from build123d import *

# Parameters (mm, degrees)
CROQUIS1_R              = 1.625
CUERPO_INICIAL_DEPTH    = 2.5
SALIENTE_EXTRUIR2_DEPTH = 195
CROQUIS6_W              = 143
CROQUIS6_H              = 28
CORTAR_EXTRUIR1_DEPTH   = 10


with BuildPart() as part:
    # Croquis1 → Cuerpo Inicial (new body)
    with BuildSketch(Plane(origin=(0, 0, 0), x_dir=(1, 0, 0), z_dir=(0, 1, 0))):
        Polygon((-71.5, -25), (-71.5, -61), (71.5, -61), (71.5, -25), (97.5, -25), (97.5, 0), (97.5, 1), (97.5, 5.7), (45, 5.7), (-45, 5.7), (-97.5, 5.7), (-97.5, 1), (-97.5, 0), (-97.5, -25), align=None)
        with Locations((-92.5, -12)):
            Circle(CROQUIS1_R, mode=Mode.SUBTRACT)
        with Locations((-64, -12)):
            Circle(CROQUIS1_R, mode=Mode.SUBTRACT)
        with Locations((-92.5, -0.46)):
            Circle(CROQUIS1_R, mode=Mode.SUBTRACT)
        with Locations((-64, -0.46)):
            Circle(CROQUIS1_R, mode=Mode.SUBTRACT)
        with Locations((64, -12)):
            Circle(CROQUIS1_R, mode=Mode.SUBTRACT)
        with Locations((92.5, -12)):
            Circle(CROQUIS1_R, mode=Mode.SUBTRACT)
        with Locations((64, -0.46)):
            Circle(CROQUIS1_R, mode=Mode.SUBTRACT)
        with Locations((92.5, -0.46)):
            Circle(CROQUIS1_R, mode=Mode.SUBTRACT)
    extrude(amount=CUERPO_INICIAL_DEPTH)

    # Croquis3 → Saliente-Extruir2 (add)
    with BuildSketch(Plane(origin=(97.5, 0, 0), x_dir=(0, 0, -1), z_dir=(1, 0, 0))):
        Polygon((5.7, 2.5), (17.833199952, 2.5), (20.75, 0), (5.7, 0), align=None)
    extrude(amount=-SALIENTE_EXTRUIR2_DEPTH)

    # Croquis6 → Cortar-Extruir1 (cut)
    with BuildSketch(Plane(origin=(0, 2.5, 0), x_dir=(1, 0, 0), z_dir=(0, 1, 0))):
        with Locations((0, -47)):
            Rectangle(CROQUIS6_W, CROQUIS6_H)
    extrude(amount=-CORTAR_EXTRUIR1_DEPTH, mode=Mode.SUBTRACT)


solid = part.part
Source: CAD feature listing. Evaluate the final solid. Frame: model axes, mm. Round coordinates to 2 decimals unless told otherwise and drop trailing zeros. Order: outer loops, then holes, each group sorted by start corner. A loop starts at its lowest first (then second) coordinate and runs counter-clockwise, first axis right, second up. Notation, with made-up numbers: (69.5, 57.25) - (128.5, 57.25) arc R20 cw to (128.5, 78.25) - close; hole circle Ø11 at (-4, 28.25). An arc over 180 degrees is marked (long way). Use a Markdown table: item, result. Add a question column.
1. Mould query, pull axis X, two halves, no side actions, for faces 1 (the cylindrical face through (-62.45, 1.23, -0.03)), 2 (the flat face through (1, 0, 6)). Classes: +X half, -X half, draft (parallel to the pull), parting line (faces both ways), or undercut.
2. Section query A-A (z = 0.46). Return the cut outline in (x, y) (3 decimals).
3. Section query C-C (y = 2). Give the number of separate pieces and of enclosed holes in the cut face, then the cut area to 3 significant figures.
4. First-contact query: pin 1 (1.2 mm diameter, centred on x = 83, y = 1.5, fed in from +Z); pin 2 (0.8 mm diameter, centred on y = 0.5, z = 27.5, fed in from +X). Flat tips, straight axial feed; report the tip coordinate or a pass-through.
5. Section query D-D (x = -92.5). Return the cut outline in (y, z) (3 decimals).
6. Section query B-B (x = 64). Return the cut outline in (y, z) (3 decimals).
7. Line query: probe 1 along X at (y, z) = (1.1, 12) (3 decimals); probe 2 along Z at (x, y) = (-92.5, 0.9) (3 decimals); probe 3 along Z at (x, y) = (64, 1.65) (3 decimals). Output: solid intervals per line, ascending.
Derived:
| question | item | result |
|---|---|---|
| 1 | face 1 | undercut |
| 1 | face 2 | draft |
| 2 | outline | (-97.5, 0) - (-94.125, 0) - (-94.125, 2.5) - (-97.5, 2.5) - close; (-90.875, 0) - (-65.625, 0) - (-65.625, 2.5) - (-90.875, 2.5) - close; (-62.375, 0) - (62.375, 0) - (62.375, 2.5) - (-62.375, 2.5) - close; (65.625, 0) - (90.875, 0) - (90.875, 2.5) - (65.625, 2.5) - close; (94.125, 0) - (97.5, 0) - (97.5, 2.5) - (94.125, 2.5) - close |
| 3 | separate pieces | 1 |
| 3 | enclosed holes | 8 |
| 3 | area | 9,540 mm2 |
| 4 | pin 1 | z = 25 |
| 4 | pin 2 | x = 71.5 |
| 5 | outline | (0, -20.75) - (2.5, -17.833) - (2.5, -1.165) - (0, -1.165) - close; (0, 2.085) - (2.5, 2.085) - (2.5, 10.375) - (0, 10.375) - close; (0, 13.625) - (2.5, 13.625) - (2.5, 25) - (0, 25) - close |
| 6 | outline | (0, -20.75) - (2.5, -17.833) - (2.5, -1.165) - (0, -1.165) - close; (0, 2.085) - (2.5, 2.085) - (2.5, 10.375) - (0, 10.375) - close; (0, 13.625) - (2.5, 13.625) - (2.5, 33) - (0, 33) - close |
| 7 | probe 1 | -97.5 to -94.125, -90.875 to -65.625, -62.375 to 62.375, 65.625 to 90.875, 94.125 to 97.5 |
| 7 | probe 2 | -19.7 to -1.165, 2.085 to 10.375, 13.625 to 25 |
| 7 | probe 3 | -18.825 to -1.165, 2.085 to 10.375, 13.625 to 33 |
